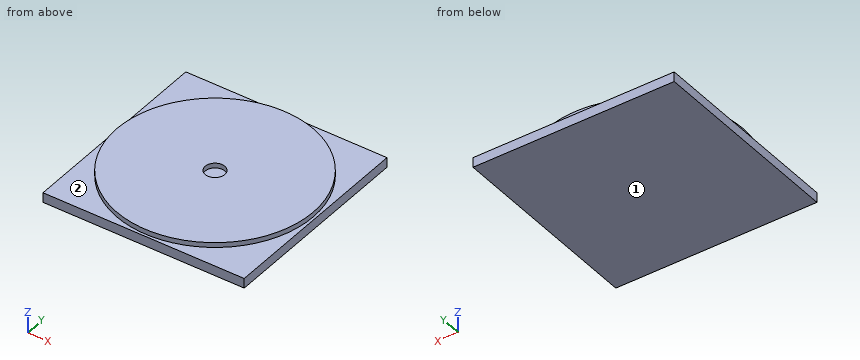
```python
from build123d import *

# Parameters (mm, degrees)
SKETCH1_W           = 41
SKETCH1_H           = 41
BOSS_EXTRUDE1_DEPTH = 2
SKETCH2_R           = 20
BOSS_EXTRUDE2_DEPTH = 1
SKETCH3_R           = 2
CUT_EXTRUDE1_DEPTH  = 1


with BuildPart() as part:
    # Sketch1 → Boss-Extrude1 (new body)
    with BuildSketch(Plane.XY):
        with Locations((-1.555803571, -8.602678571)):
            Rectangle(SKETCH1_W, SKETCH1_H)
    extrude(amount=BOSS_EXTRUDE1_DEPTH)

    # Sketch2 → Boss-Extrude2 (add)
    with BuildSketch(Plane.XY.offset(2)):
        with Locations((-1.555803571, -8.602678571)):
            Circle(SKETCH2_R)
    extrude(amount=BOSS_EXTRUDE2_DEPTH)

    # Sketch3 → Cut-Extrude1 (cut)
    with BuildSketch(Plane.XY.offset(3)):
        with Locations((-1.555803571, -8.602678571)):
            Circle(SKETCH3_R)
    extrude(amount=-CUT_EXTRUDE1_DEPTH, mode=Mode.SUBTRACT)


solid = part.part
```
Work out the finished part from the listing and answer in its coordinate system (mm). Face numbers are marked on the shaded views. A direction names the side the tool comes from. Give positions to 0.01 mm unless a question says otherwise; leave off trailing zeros. Write each loop counter-clockwise with the first axis right and the second up, starting at its lowest first coordinate (ties: lowest second). Pieces come first, ordered by that corner, then holes.
(1) The part is cut by section A-A on x = 6. Write down the section's boundary in (y, z), plus the area to 3 significant figures.
Final values:
outline: (-29.1, 0) - (11.9, 0) - (11.9, 2) - (9.92, 2) - (9.92, 3) - (-27.12, 3) - (-27.12, 2) - (-29.1, 2) - close
area: 119 mm2
(2) The part is cut by section C-C on x = -1.5. Write down the section's boundary in (y, z).
Final values:
outline: (-29.1, 0) - (11.9, 0) - (11.9, 2) - (11.4, 2) - (11.4, 3) - (-6.6, 3) - (-6.6, 2) - (-10.6, 2) - (-10.6, 3) - (-28.6, 3) - (-28.6, 2) - (-29.1, 2) - close
(3) A flat-ended cylindrical pin translates along its axis: pin 1 Ø2 at (x, y) = (-2.5, -8.5) entering from +Z. Find the tip coordinate at first contact, or state that the pin passes through.
Final values:
pin 1: stops at z = 2
(4) Which of the six approach directions +Z, -Z, +X, -X, +Y, -Y give full straight-line access (tool end or side, diameter ignored) to the marked faces 1 and 2?
Final values:
face 1: -Z, +X, -X, +Y, -Y
face 2: +Z
(5) The part is cut by section B-B on y = -13. Write down the section's boundary in (x, z), plus the area to 3 significant figures.
Final values:
outline: (-22.06, 0) - (18.94, 0) - (18.94, 2) - (17.95, 2) - (17.95, 3) - (-21.07, 3) - (-21.07, 2) - (-22.06, 2) - close
area: 121 mm2
(6) Straight lines are drawn through the part: line 1 (Z direction, x = -19, y = -21.5); line 2 (Y direction, x = -19, z = 2.6); line 3 (X direction, y = -2.5, z = 2.3). For each, find the intervals that lie inside material, in ascending order.
Final values:
line 1: z = 0 to 2
line 2: y = -18.39 to 1.18
line 3: x = -20.6 to 17.49
